from build123d import *

# Parameters (mm, degrees)
SKETCH2_R           = 1.4
SKETCH2_R_2         = 0.45
SKETCH2_R_3         = 0.5
BOSS_EXTRUDE1_DEPTH = 1.7


with BuildPart() as part:
    # Sketch2 → Boss-Extrude1 (new body)
    with BuildSketch(Plane.XY):
        with BuildLine():
            Line((29.5, 28.25), (-29.5, 28.25))
            ThreePointArc((-29.5, 28.25), (-31.621320344, 27.371320344), (-32.5, 25.25))
            Line((-32.5, 25.25), (-32.5, 8.25))
            Line((-32.5, 8.25), (-28.5, 8.25))
            ThreePointArc((-28.5, 8.25), (-27.792893219, 7.957106781), (-27.5, 7.25))
            Line((-27.5, 7.25), (-27.5, -7.75))
            ThreePointArc((-27.5, -7.75), (-27.792893219, -8.457106781), (-28.5, -8.75))
            Line((-28.5, -8.75), (-32.4, -8.75))
            Line((-32.4, -8.75), (-32.5, -25.25))
            ThreePointArc((-32.5, -25.25), (-31.626652319, -27.376652319), (-29.5, -28.25))
            Line((-29.5, -28.25), (29.5, -28.25))
            ThreePointArc((29.5, -28.25), (31.621320344, -27.371320344), (32.5, -25.25))
            Line((32.5, -25.25), (32.5, 25.25))
            ThreePointArc((32.5, 25.25), (31.621320344, 27.371320344), (29.5, 28.25))
        make_face()
        with Locations((-29, -24.75)):
            Circle(SKETCH2_R, mode=Mode.SUBTRACT)
        with Locations((-29, 24.25)):
            Circle(SKETCH2_R, mode=Mode.SUBTRACT)
        with Locations((29, 24.25)):
            Circle(SKETCH2_R, mode=Mode.SUBTRACT)
        with Locations((29, -24.75)):
            Circle(SKETCH2_R, mode=Mode.SUBTRACT)
        with Locations((-24.13, 25.52)):
            Circle(SKETCH2_R_2, mode=Mode.SUBTRACT)
        with Locations((-21.59, 25.52)):
            Circle(SKETCH2_R_2, mode=Mode.SUBTRACT)
        with Locations((-19.05, 25.52)):
            Circle(SKETCH2_R_2, mode=Mode.SUBTRACT)
        with Locations((-16.51, 25.52)):
            Circle(SKETCH2_R_2, mode=Mode.SUBTRACT)
        with Locations((-13.97, 25.52)):
            Circle(SKETCH2_R_2, mode=Mode.SUBTRACT)
        with Locations((-11.43, 25.52)):
            Circle(SKETCH2_R_2, mode=Mode.SUBTRACT)
        with Locations((-8.89, 25.52)):
            Circle(SKETCH2_R_2, mode=Mode.SUBTRACT)
        with Locations((-6.35, 25.52)):
            Circle(SKETCH2_R_2, mode=Mode.SUBTRACT)
        with Locations((-3.81, 25.52)):
            Circle(SKETCH2_R_2, mode=Mode.SUBTRACT)
        with Locations((-1.27, 25.52)):
            Circle(SKETCH2_R_2, mode=Mode.SUBTRACT)
        with Locations((1.27, 25.52)):
            Circle(SKETCH2_R_2, mode=Mode.SUBTRACT)
        with Locations((3.81, 25.52)):
            Circle(SKETCH2_R_2, mode=Mode.SUBTRACT)
        with Locations((6.35, 25.52)):
            Circle(SKETCH2_R_2, mode=Mode.SUBTRACT)
        with Locations((8.89, 25.52)):
            Circle(SKETCH2_R_2, mode=Mode.SUBTRACT)
        with Locations((11.43, 25.52)):
            Circle(SKETCH2_R_2, mode=Mode.SUBTRACT)
        with Locations((13.97, 25.52)):
            Circle(SKETCH2_R_2, mode=Mode.SUBTRACT)
        with Locations((16.51, 25.52)):
            Circle(SKETCH2_R_2, mode=Mode.SUBTRACT)
        with Locations((19.05, 25.52)):
            Circle(SKETCH2_R_2, mode=Mode.SUBTRACT)
        with Locations((21.59, 25.52)):
            Circle(SKETCH2_R_2, mode=Mode.SUBTRACT)
        with Locations((24.13, 25.52)):
            Circle(SKETCH2_R_2, mode=Mode.SUBTRACT)
        with Locations((-21.59, 22.98)):
            Circle(SKETCH2_R_2, mode=Mode.SUBTRACT)
        with Locations((-19.05, 22.98)):
            Circle(SKETCH2_R_2, mode=Mode.SUBTRACT)
        with Locations((-16.51, 22.98)):
            Circle(SKETCH2_R_2, mode=Mode.SUBTRACT)
        with Locations((-13.97, 22.98)):
            Circle(SKETCH2_R_2, mode=Mode.SUBTRACT)
        with Locations((-11.43, 22.98)):
            Circle(SKETCH2_R_2, mode=Mode.SUBTRACT)
        with Locations((-8.89, 22.98)):
            Circle(SKETCH2_R_2, mode=Mode.SUBTRACT)
        with Locations((-6.35, 22.98)):
            Circle(SKETCH2_R_2, mode=Mode.SUBTRACT)
        with Locations((-3.81, 22.98)):
            Circle(SKETCH2_R_2, mode=Mode.SUBTRACT)
        with Locations((-1.27, 22.98)):
            Circle(SKETCH2_R_2, mode=Mode.SUBTRACT)
        with Locations((1.27, 22.98)):
            Circle(SKETCH2_R_2, mode=Mode.SUBTRACT)
        with Locations((3.81, 22.98)):
            Circle(SKETCH2_R_2, mode=Mode.SUBTRACT)
        with Locations((6.35, 22.98)):
            Circle(SKETCH2_R_2, mode=Mode.SUBTRACT)
        with Locations((8.89, 22.98)):
            Circle(SKETCH2_R_2, mode=Mode.SUBTRACT)
        with Locations((11.43, 22.98)):
            Circle(SKETCH2_R_2, mode=Mode.SUBTRACT)
        with Locations((13.97, 22.98)):
            Circle(SKETCH2_R_2, mode=Mode.SUBTRACT)
        with Locations((16.51, 22.98)):
            Circle(SKETCH2_R_2, mode=Mode.SUBTRACT)
        with Locations((19.05, 22.98)):
            Circle(SKETCH2_R_2, mode=Mode.SUBTRACT)
        with Locations((21.59, 22.98)):
            Circle(SKETCH2_R_2, mode=Mode.SUBTRACT)
        with Locations((24.13, 22.98)):
            Circle(SKETCH2_R_2, mode=Mode.SUBTRACT)
        with Locations((-24.13, 22.98)):
            Circle(SKETCH2_R_2, mode=Mode.SUBTRACT)
        with Locations((-23.498, -24.567)):
            Circle(SKETCH2_R_3, mode=Mode.SUBTRACT)
        with Locations((-19.998, -24.567)):
            Circle(SKETCH2_R_3, mode=Mode.SUBTRACT)
        with Locations((-16.498, -24.567)):
            Circle(SKETCH2_R_3, mode=Mode.SUBTRACT)
        with Locations((-12.998, -24.567)):
            Circle(SKETCH2_R_3, mode=Mode.SUBTRACT)
        with Locations((-9.498, -24.567)):
            Circle(SKETCH2_R_3, mode=Mode.SUBTRACT)
        with Locations((-4.829, -24.567)):
            Circle(SKETCH2_R_3, mode=Mode.SUBTRACT)
        with Locations((-1.329, -24.567)):
            Circle(SKETCH2_R_3, mode=Mode.SUBTRACT)
        with Locations((2.171, -24.567)):
            Circle(SKETCH2_R_3, mode=Mode.SUBTRACT)
        with Locations((5.671, -24.567)):
            Circle(SKETCH2_R_3, mode=Mode.SUBTRACT)
        with Locations((9.171, -24.567)):
            Circle(SKETCH2_R_3, mode=Mode.SUBTRACT)
        with Locations((18.505, -24.567)):
            Circle(SKETCH2_R_3, mode=Mode.SUBTRACT)
        with Locations((22.005, -24.567)):
            Circle(SKETCH2_R_3, mode=Mode.SUBTRACT)
        with BuildLine():
            Line((13.5, -9.25), (13.5, -24.25))
            ThreePointArc((13.5, -24.25), (12.5, -25.25), (11.5, -24.25))
            Line((11.5, -24.25), (11.5, -9.25))
            ThreePointArc((11.5, -9.25), (12.5, -8.25), (13.5, -9.25))
        make_face(mode=Mode.SUBTRACT)
    extrude(amount=BOSS_EXTRUDE1_DEPTH)


solid = part.part
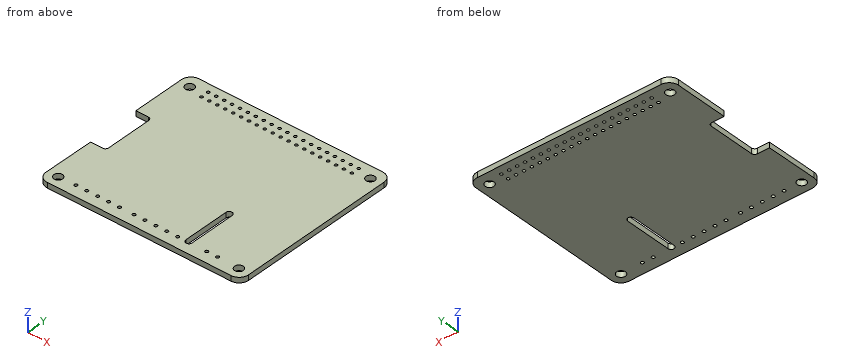
Verification items for the finished model (mm, model axes). Round coordinates to 2 decimals unless told otherwise and drop trailing zeros. Loops run counter-clockwise (first coordinate to the right, second up) from the corner with the lowest first, then second, coordinate; pieces in that order, holes last. Notation, with made-up numbers: (21.5, -22) - (47.5, -22) arc R20 cw to (47.5, -8) - close; hole circle Ø10 at (-31.75, 39.25). An arc over 180 degrees is marked (long way). Use a Markdown table: item, result. Add a question column.
1. Gauge pin test, flat ends, axial feed: pin 1 (0.5 mm diameter, centred on x = -31, z = 1, fed in from +Y); pin 2 (1 mm diameter, centred on y = 4, z = 0.5, fed in from -X); pin 3 (4.5 mm diameter, centred on x = 29, y = 24.25, fed in from +Z). Record the tip position at first contact, or that the pin passes through.
2. Section check B-B, the plane y = -13. Record the boundary of the cut face in (x, z), plus the area to 3 significant figures.
3. Section check C-C, the plane y = -7. Record the boundary of the cut face in (x, z), plus the area to 3 significant figures.
4. Thickness scan on probe 1 along Y at (x, z) = (-29, 1); probe 2 along Y at (x, z) = (19.05, 0.6); probe 3 along Y at (x, z) = (-28, 1.35). Record the ranges inside material, lowest first. Write a range as [from, to].
5. Section check A-A, the plane y = 24.25. Record the boundary of the cut face in (x, z).
Checks:
| question | item | result |
|---|---|---|
| 1 | pin 1 | stops at y = 27.98 |
| 1 | pin 2 | stops at x = -27.5 |
| 1 | pin 3 | stops at z = 1.7 |
| 2 | outline | (-32.43, 0) - (11.5, 0) - (11.5, 1.7) - (-32.43, 1.7) - close; (13.5, 0) - (32.5, 0) - (32.5, 1.7) - (13.5, 1.7) - close |
| 2 | area | 107 mm^2 |
| 3 | outline | (-27.5, 0) - (32.5, 0) - (32.5, 1.7) - (-27.5, 1.7) - close |
| 3 | area | 102 mm^2 |
| 4 | probe 1 | y = [-28.25, -26.15], [-23.35, -8.75], [8.25, 22.85], [25.65, 28.25] |
| 4 | probe 2 | y = [-28.25, 22.53], [23.43, 25.07], [25.97, 28.25] |
| 4 | probe 3 | y = [-28.25, -25.73], [-23.77, -8.62], [8.12, 23.27], [25.23, 28.25] |
| 5 | outline | (-32.5, 0) - (-30.4, 0) - (-30.4, 1.7) - (-32.5, 1.7) - close; (-27.6, 0) - (27.6, 0) - (27.6, 1.7) - (-27.6, 1.7) - close; (30.4, 0) - (32.5, 0) - (32.5, 1.7) - (30.4, 1.7) - close |
